Build history of the part. All positions in model axes, mm. Give positions to 0.01 mm unless a question says otherwise; leave off trailing zeros. Order: outer loops, then holes, each group sorted by start corner. A loop starts at its lowest first (then second) coordinate and runs counter-clockwise, first axis right, second up. Notation, with made-up numbers: (7.25, 18) - (44.25, 18) arc R25 cw to (44.25, 55) - close; hole circle Ø9 at (11, 76.25). An arc over 180 degrees is marked (long way). Write each question's results on one line, items separated by ' | '. Start each with the question number.
1) Cut at A-A on z = 3. List the corners of the cut face in (x, y).
2) Two-plate mould, pull along Y, no slides. Class faces 1 (the face through (-0.38, 34.1, -39.14)), 2 (the face through (-29.37, 6.69, -0.52)), 3 (the face through (-29.34, 28.27, -0.52)), 4 (the face through (-30, 2, 1)): +Y half, -Y half, draft (parallel to the pull), parting line (faces both ways), or undercut.
3) Drill centre lines: line 1 along Y through (x, z) = (-27, -24.5); line 2 along X through (y, z) = (18, 25.5); line 3 along Y through (x, z) = (-24.5, -4.5). Where is each one in solid material? Low to high. Write a range as from..to.
from build123d import *

# Parameters (mm, degrees)
EXTRUDE_1_DEPTH = 40
FILLET_1_R      = 3
FILLET_2_R      = 3


with BuildPart() as part:
    # Эскиз1 → Бобышка-Вытянуть1 (new, symmetric)
    with BuildSketch(Plane.XY):
        with BuildLine():
            Line((-30, 0), (30, 0))
            Line((30, 0), (30, 7.5))
            ThreePointArc((30, 7.5), (20, 17.5), (30, 27.5))
            Line((30, 27.5), (30, 35))
            Line((30, 35), (-30, 35))
            Line((-30, 35), (-30, 27.5))
            ThreePointArc((-30, 27.5), (-20, 17.5), (-30, 7.5))
            Line((-30, 7.5), (-30, 0))
        make_face()
    extrude(amount=EXTRUDE_1_DEPTH, both=True)

    # Скругление1
    fillet_1_edges = [part.edges().sort_by_distance(p)[0] for p in [
        (-30, 7.5, 0),
        (-30, 27.5, 0),
        (-30, 35, 0),
        (30, 35, 0),
        (30, 27.5, 0),
        (30, 7.5, 0),
    ]]
    fillet(fillet_1_edges, radius=FILLET_1_R)

    # Скругление2
    fillet_2_edges = [part.edges().sort_by_distance(p)[0] for p in [
        (30, 2.42544468, 40),
        (20, 17.5, -40),
        (20, 17.5, 40),
        (-30, 2.42544468, -40),
        (-20, 17.5, -40),
        (-30, 31.07455532, -40),
        (0, 35, -40),
        (30, 31.07455532, -40),
        (29.121320344, 34.121320344, -40),
        (-29.121320344, 34.121320344, -40),
        (29.353393622, 28.288589622, -40),
        (-29.353393622, 28.288589622, -40),
        (-29.353393622, 6.711410378, -40),
        (29.353393622, 6.711410378, -40),
        (-30, 2.42544468, 40),
        (30, 31.07455532, 40),
        (0, 35, 40),
        (-30, 31.07455532, 40),
        (-20, 17.5, 40),
        (29.121320344, 34.121320344, 40),
        (-29.121320344, 34.121320344, 40),
        (29.353393622, 28.288589622, 40),
        (-29.353393622, 28.288589622, 40),
        (-29.353393622, 6.711410378, 40),
        (29.353393622, 6.711410378, 40),
        (30, 2.42544468, -40),
    ]]
    fillet(fillet_2_edges, radius=FILLET_2_R)


solid = part.part
Results:
1) outline: (-30, 0) - (30, 0) - (30, 4.85) arc R3 ccw to (27.69, 7.77) arc R10 cw to (27.69, 27.23) arc R3 ccw to (30, 30.15) - (30, 32) arc R3 ccw to (27, 35) - (-27, 35) arc R3 ccw to (-30, 32) - (-30, 30.15) arc R3 ccw to (-27.69, 27.23) arc R10 cw to (-27.69, 7.77) arc R3 ccw to (-30, 4.85) - close
2) face 1: +Y half | face 2: undercut | face 3: undercut | face 4: draft
3) line 1: 0..7.96, 27.04..35 | line 2: -20.01..20.01 | line 3: 0..9.15, 25.85..35
